```python
from build123d import *

# Parameters (mm, degrees)
SKETCH_W        = 100
SKETCH_H        = 60
PAD_DEPTH       = 16
FILLET_R        = 5
FILLET001_R     = 3
POCKET_DEPTH    = 13
SKETCH002_W     = 10
SKETCH002_H     = 1
POCKET001_DEPTH = 5
CHAMFER_1_ANGLE = 48
CHAMFER_1_SIZE  = 0.9
CHAMFER_2_ANGLE = 48
CHAMFER_2_SIZE  = 0.9
FILLET002_R     = 1


with BuildPart() as part:
    # Sketch → Pad (new body)
    with BuildSketch(Plane.XY):
        with Locations((50, 30)):
            Rectangle(SKETCH_W, SKETCH_H)
    extrude(amount=PAD_DEPTH)

    # Fillet
    fillet_edges = [part.edges().sort_by_distance(p)[0] for p in [
        (100, 0, 8),
        (100, 60, 8),
        (0, 60, 8),
        (0, 0, 8),
    ]]
    fillet(fillet_edges, radius=FILLET_R)

    # Fillet001
    fillet001_edges = [part.edges().sort_by_distance(p)[0] for p in [
        (50, 60, 0),
    ]]
    fillet(fillet001_edges, radius=FILLET001_R)

    # Sketch001 (on Face6 of Pad) → Pocket (cut)
    with BuildSketch(Plane.XY.offset(16)):
        with BuildLine():
            Line((6, 3), (94, 3))
            ThreePointArc((94, 3), (96.12132, 3.87868), (97, 6))
            Line((97, 6), (97, 54))
            ThreePointArc((97, 54), (96.12132, 56.12132), (94, 57))
            Line((94, 57), (6, 57))
            ThreePointArc((6, 57), (3.87868, 56.12132), (3, 54))
            Line((3, 54), (3, 6))
            ThreePointArc((3, 6), (3.87868, 3.87868), (6, 3))
        make_face()
    extrude(amount=-POCKET_DEPTH, mode=Mode.SUBTRACT)

    # Sketch002 (on Face4 of Pocket) → Pocket001 (cut)
    with BuildSketch(Plane.XY.offset(16)):
        with Locations((50, 0.5)):
            Rectangle(SKETCH002_W, SKETCH002_H)
        with Locations((50, 59.5)):
            Rectangle(SKETCH002_W, SKETCH002_H)
    extrude(amount=-POCKET001_DEPTH, mode=Mode.SUBTRACT)

    # Chamfer 1
    chamfer_1_edges = [part.edges().sort_by_distance(p)[0] for p in [
        (50, 59, 11),
    ]]
    chamfer_1_side = part.faces().sort_by_distance((50, 59, 13.5))[0]
    chamfer(chamfer_1_edges, length=CHAMFER_1_SIZE, angle=CHAMFER_1_ANGLE, reference=chamfer_1_side)

    # Chamfer 2
    chamfer_2_edges = [part.edges().sort_by_distance(p)[0] for p in [
        (50, 1, 11),
    ]]
    chamfer_2_side = part.faces().sort_by_distance((50, 0.5, 11))[0]
    chamfer(chamfer_2_edges, length=CHAMFER_2_SIZE, angle=CHAMFER_2_ANGLE, reference=chamfer_2_side)

    # Fillet002
    fillet002_edges = [part.edges().sort_by_distance(p)[0] for p in [
        (3, 30, 16),
    ]]
    fillet(fillet002_edges, radius=FILLET002_R)


solid = part.part
```
Here's how the part is built. I have some questions about the finished solid (model axes, mm). A direction names the side the tool comes from. Round coordinates to 2 decimals unless told otherwise and drop trailing zeros. Order: outer loops, then holes, each group sorted by start corner. A loop starts at its lowest first (then second) coordinate and runs counter-clockwise, first axis right, second up. Notation, with made-up numbers: M 53,15.5 L 88,15.5 A14 cw 88,40.5 Z; hole C 85.25,53 d11. An arc over 180 degrees is marked long. Answer in a Markdown table with one row per item.
Item 1: For faces 5 (the face through (51, 57, 9)), 6 (the face through (100, 30, 9)), 7 (the face through (35, 1, 16)), 8 (the face through (50, 1, 14)), 9 (the face through (50, 59, 14)), which set-ups out of +Z, -Z, +X, -X, +Y, -Y let a thin tool reach every point of the face, with its end or its side?
A:
| item | result |
|---|---|
| face 5 | +Z |
| face 6 | +Z, -Z, +X, +Y, -Y |
| face 7 | +Z, +X, -X, +Y, -Y |
| face 8 | +Z, -Y |
| face 9 | +Z, +Y |
Item 2: Thinking about a two-plate mould opening in Y: for faces 1 (the face through (96.14, 56.1, 9.08)), 2 (the face through (49.37, 0.9, 0.86)), 3 (the face through (99, 58, 10)), 4 (the face through (97, 30, 9)), which applies, +Y half, -Y half, draft (parallel to the pull), parting line (faces both ways), or undercut?
A:
| item | result |
|---|---|
| face 1 | undercut |
| face 2 | -Y half |
| face 3 | +Y half |
| face 4 | undercut |
Item 3: Imagine slicing it at B-B, the plane x = 42. Write out the boundary of the cut face in (y, z).
A:
| item | result |
|---|---|
| outline | M 0,3 A3 ccw 3,0 L 57,0 A3 ccw 60,3 L 60,16 L 58,16 A1 ccw 57,15 L 57,3 L 3,3 L 3,15 A1 ccw 2,16 L 0,16 Z |
Item 4: Imagine slicing it at C-C, the plane y = 39.5. Write out the boundary of the cut face in (x, z), and give its area (3 significant figures).
A:
| item | result |
|---|---|
| outline | M 0,3 A3 ccw 3,0 L 97,0 A3 ccw 100,3 L 100,16 L 98,16 A1 ccw 97,15 L 97,3 L 3,3 L 3,15 A1 ccw 2,16 L 0,16 Z |
| area | 374 mm2 |
Item 5: Imagine slicing it at A-A, the plane z = 7. Write out the boundary of the cut face in (x, y), and give its area (3 significant figures).
A:
| item | result |
|---|---|
| outline | M 0,5 A5 ccw 5,0 L 95,0 A5 ccw 100,5 L 100,55 A5 ccw 95,60 L 5,60 A5 ccw 0,55 Z; hole M 3,6 A3 ccw 6,3 L 94,3 A3 ccw 97,6 L 97,54 A3 ccw 94,57 L 6,57 A3 ccw 3,54 Z |
| area | 910 mm2 |
Item 6: If I drill on L1, parallel to X at y = 49.5, z = 10; L2, parallel to Y at x = 8, z = 10; L3, parallel to Z at x = 21, y = 14.5, over which ranges is the centre line in solid material (lowest first)? Write a range as from..to.
A:
| item | result |
|---|---|
| L1 | x = 0..3, 97..100 |
| L2 | y = 0..3, 57..60 |
| L3 | z = 0..3 |
Item 7: I'm going to push flat-ended pins straight in: pin 1 (1.1 mm diameter, centred on y = 0.5, z = 13, fed in from +X); pin 2 (1.1 mm diameter, centred on y = 0.5, z = 13, fed in from -X); pin 3 (0.5 mm diameter, centred on y = 59.5, z = 14, fed in from -X). Where does each tip first touch, or does it pass through?
A:
| item | result |
|---|---|
| pin 1 | stops at x = 98.07 |
| pin 2 | stops at x = 1.93 |
| pin 3 | stops at x = 2.37 |
